Check sheet for the modelled part. Datum: model origin and axes. Units: mm. A direction names the side the tool comes from. Round coordinates to 2 decimals unless told otherwise and drop trailing zeros. Write each loop counter-clockwise with the first axis right and the second up, starting at its lowest first coordinate (ties: lowest second). Pieces come first, ordered by that corner, then holes. Notation, with made-up numbers: (59, 88) -> (81, 88) arc R19 ccw to (81, 98) -> close; hole circle Ø2 at (-30, 45.25). An arc over 180 degrees is marked (long way). Use one line per item in the form item = value. Start each with the question number.
```python
from build123d import *

# Parameters (mm, degrees)
F0_R      = 5.45168
F1_DEPTH  = 5.08
F2_R      = 3.834329
F3_DEPTH  = 25.4
F4_R      = 32.422249
F5_DEPTH  = 5.08
F6_W      = 36.716256
F6_H      = 65.308068
F7_DEPTH  = 5.08
F9_W      = 4.441859
F9_H      = 27.334548
F9_W_2    = 4.413207
F9_H_2    = 27.691893
F9_W_3    = 5.325806
F9_H_3    = 27.507089
F10_DEPTH = 25.4
F12_DEPTH = 25.4
F14_DEPTH = 25.4


with BuildPart() as f1:
    # F0 (on Top) → F1 (new body)
    with BuildSketch(Plane.XY):
        Circle(F0_R)
    extrude(amount=F1_DEPTH)

    # F2 (on face) → F3 (cut)
    with BuildSketch(Plane.XY.offset(5.08)):
        Circle(F2_R)
    extrude(amount=-F3_DEPTH, mode=Mode.SUBTRACT)

    # F4 (on Top) → F5 (join)
    with BuildSketch(Plane.XY):
        with Locations((0, -35.921536)):
            Circle(F4_R)
    extrude(amount=F5_DEPTH)

    # F6 (on Top) → F7 (join)
    with BuildSketch(Plane.XY):
        with Locations((-0.742003, -76.719692)):
            Rectangle(F6_W, F6_H)
    extrude(amount=F7_DEPTH)

    # F9 (on face) → F10 (cut)
    with BuildSketch(Plane.XY.offset(5.08)):
        with Locations((-11.158781, -91.761265)):
            Rectangle(F9_W, F9_H)
        with Locations((-1.842302, -91.582593)):
            Rectangle(F9_W_2, F9_H_2)
        with Locations((8.863835, -91.674994)):
            Rectangle(F9_W_3, F9_H_3)
    extrude(amount=-F10_DEPTH, mode=Mode.SUBTRACT)

    # F11 (on face) → F12 (cut)
    with BuildSketch(Plane.XY.offset(5.08)):
        Polygon((9.909331, -59.593312), (4.586765, -48.460342), (5.977736, -67.931563), align=None)
        Polygon((-8.305341, -58.362357), (-2.982776, -69.495328), (-4.373746, -50.024107), align=None)
    extrude(amount=-F12_DEPTH, mode=Mode.SUBTRACT)

    # F13 (on face) → F14 (cut)
    with BuildSketch(Plane.XY.offset(5.08)):
        Polygon((23.395628, -22.520874), (3.782702, -43.190122), (7.484366, -44.308007), (23.395628, -37.764173), align=None)
        Polygon((0, -43.190122), (-22.690315, -20.113243), (-22.690315, -35.91549), align=None)
    extrude(amount=-F14_DEPTH, mode=Mode.SUBTRACT)


solid = f1.part
```
1. Sectioned sample at C-C (y = -90). Enter the section's corners in (x, z), and give its area (3 significant figures).
2. Depth check by flat-ended pin: pin 1 (2 mm diameter, centred on y = -82.5, z = 2.5, fed in from +X); pin 2 (1.5 mm diameter, centred on y = -29, z = 2.5, fed in from +X); pin 3 (1.5 mm diameter, centred on y = -30.5, z = 3.5, fed in from -X). Enter the tip coordinate at first touch or a pass-through.
3. Scan lines: probe 1 along X at (y, z) = (-97.5, 2.4); probe 2 along X at (y, z) = (-57, 0.4); probe 3 along Y at (x, z) = (-8, 1.6). Record each from-to range of solid material in increasing order.
4. Sectioned sample at D-D (x = -14.5). Enter the section's corners in (y, z), and give its area (3 significant figures).
5. Mould release check, pull along Y, two halves, no side actions. Record for faces 3 (the face through (17.616, -87, 3)), 4 (the face through (-22.69, -28, 3)): +Y half, -Y half, draft (parallel to the pull), parting line (faces both ways), or undercut.
6. Sectioned sample at B-B (z = 1.5). Give the number of separate pieces and of enclosed holes in the cut face, and give its area (3 significant figures).
7. Sectioned sample at A-A (y = 0). Enter the section's corners in (x, z), and give its area (3 significant figures).
8. Tool access check on faces 1 (the face through (0, -51, 5.08)), 2 (the face through (-11.504, -39.502, 2.576)). Record the directions out of +Z, -Z, +X, -X, +Y, -Y that give a thin tool (end or side, any length) a straight path to the whole face; none if there is none.
Returned:
q1.outline = (-19.1, 0) -> (-13.38, 0) -> (-13.38, 5.08) -> (-19.1, 5.08) -> close; (-8.94, 0) -> (-4.05, 0) -> (-4.05, 5.08) -> (-8.94, 5.08) -> close; (0.36, 0) -> (6.2, 0) -> (6.2, 5.08) -> (0.36, 5.08) -> close; (11.53, 0) -> (17.62, 0) -> (17.62, 5.08) -> (11.53, 5.08) -> close
q1.area = 114 mm^2
q2.pin_1 = 17.62
q2.pin_2 = 31.83
q2.pin_3 = -32.08
q3.probe_1 = -19.1 to -13.38, -8.94 to -4.05, 0.36 to 6.2, 11.53 to 17.62
q3.probe_2 = -24.64 to -7.66, -3.88 to 5.2, 8.67 to 24.64
q3.probe_3 = -109.37 to -59, -57.71 to -40.63, -35.05 to -4.5
q4.outline = (-109.37, 0) -> (-38.54, 0) -> (-38.54, 5.08) -> (-109.37, 5.08) -> close; (-28.44, 0) -> (-6.92, 0) -> (-6.92, 5.08) -> (-28.44, 5.08) -> close
q4.area = 469 mm^2
q5.face_3 = draft
q5.face_4 = undercut
q6.separate_pieces = 1
q6.enclosed_holes = 8
q6.area = 4,090 mm^2
q7.outline = (-5.45, 0) -> (-3.83, 0) -> (-3.83, 5.08) -> (-5.45, 5.08) -> close; (3.83, 0) -> (5.45, 0) -> (5.45, 5.08) -> (3.83, 5.08) -> close
q7.area = 16.4 mm^2
q8.face_1 = +Z, +X, -X, +Y, -Y
q8.face_2 = +Z, -Z
